Autodesk Inventor part; units mm, degrees
ref_plane "YZ Plane" through (0, 0, 0) normal (1, 0, 0) x (0, 1, 0)
ref_plane "XZ Plane" through (0, 0, 0) normal (0, 1, 0) x (-1, 0, 0)
ref_plane "XY Plane" through (0, 0, 0) normal (0, 0, 1) x (1, 0, 0)
sketch "Sketch1" plane through (0, 0, 0) normal (0, 0, 1) x (1, 0, 0)
  line L0 (-28, 11) -> (28, 11)
  line L1 (28, 11) -> (28, 9)
  line L2 (28, 9) -> (-28, 9)
  line L3 (-28, 9) -> (-28, 11)
  line L4 (-27, -7) -> (27, -7)
  line L5 (27, -7) -> (27, -9)
  line L6 (27, -9) -> (-27, -9)
  line L7 (-27, -9) -> (-27, -7)
  line L8 (-20, 1.5) -> (20, 1.5)
  line L9 (20, 1.5) -> (20, -1.5)
  line L10 (20, -1.5) -> (-20, -1.5)
  line L11 (-20, -1.5) -> (-20, 1.5)
  line L12 (26.5, 11) -> (27.8333, 15)
  line L13 (27.8333, 15) -> (29.3333, 15)
  line L14 (29.3333, 15) -> (29.3333, 4.5)
  line L15 (29.3333, 4.5) -> (22.8333, 0)
  line L16 (22.8333, 0) -> (29, -6.1667)
  line L17 (29, -6.1667) -> (29, -13)
  line L18 (29, -13) -> (27.5, -13)
  line L19 (27.5, -13) -> (25.5, -9)
  line L20 (20, -1.5) -> (25.5, -7)
  line L21 (26.5, 9) -> (28, 9)
  line L22 (28, 9) -> (28, 11)
  line L23 (28, 11) -> (26.5, 11)
  line L24 (26.5, 9) -> (26.5, 6)
  line L25 (26.5, 6) -> (20, 1.5)
  point P0 (0, 0)
  point P1 (0, 9)
  point P2 (0, -7)
  point P3 (0, -1.5)
  point P4 (20, 0)
  dimension "d0" = 2
  dimension "d1" = 2
  dimension "d2" = 56
  dimension "d3" = 54
  dimension "d4" = 7
  dimension "d6" = 3
  dimension "d7" = 40
  dimension "d8" = 1.5
  dimension "d9" = 1.5
  dimension "d10" = 1.5
  dimension "d11" = 1.5
  dimension "d13" = 2
  dimension "d14" = 1.5
  dimension "d16" = 4
  dimension "d17" = 4
  dimension "d18" = 1.5
  dimension "d26" = 3
  dimension "d28" = 15
extrude "Extrusion1" add sketch "Sketch1" along normal blind 7 contours L12 L13 L14 L15 L16 L17 L18 L19 L6 L5 L4 L20 L9 L25 L24 L2 L1 L0
mirror "Mirror1" about plane through (0, 0, 0) normal (1, 0, 0) of "Extrusion1"
sketch "Sketch2" plane through (0, 0, 0) normal (0, 0, 1) x (1, 0, 0)
  line L0 (-20, 1.5) -> (-20, -1.5)
  line L1 (20, 1.5) -> (20, -1.5)
  line L2 (-20, 1.5) -> (20, 1.5)
  line L3 (20, 1.5) -> (20, -1.5)
  line L4 (20, -1.5) -> (-20, -1.5)
  line L5 (-20, -1.5) -> (-20, 1.5)
  point P0 (0, 0)
extrude "Extrusion2" add sketch "Sketch2" along normal up to surface (7 mm away)
fillet "Fillet1" radius 2 6 edges at (22.8333, 0, 3.5) (-22.8333, 0, 3.5) (-29.3333, 4.5, 3.5) (29.3333, 4.5, 3.5) (29, -6.1667, 3.5) (-29, -6.1667, 3.5)
fillet "Fillet2" radius 1 4 edges at (-26.5, 9, 3.5) (26.5, 9, 3.5) (25.5, -7, 3.5) (-25.5, -7, 3.5)
fillet "Fillet3" radius 0.5 4 edges at (-26.5, 11, 3.5) (26.5, 11, 3.5) (25.5, -9, 3.5) (-25.5, -9, 3.5)
fillet "Fillet4" radius 2 2 edges at (26.5, 6, 3.5) (-26.5, 6, 3.5)
properties part number "conector-rpi-arduino-improved"
Read the model definition and answer for the solid it produces. Units are mm, in the model's axes. A direction names the side the tool comes from. Give positions to 0.01 mm unless a question says otherwise; leave off trailing zeros. Write each loop counter-clockwise with the first axis right and the second up, starting at its lowest first coordinate (ties: lowest second). Pieces come first, ordered by that corner, then holes. Notation, with made-up numbers: (40, 40) -> (96, 40) arc R35 ccw to (96, 77) -> close; hole circle Ø3 at (37.5, -34). An arc over 180 degrees is marked (long way). Answer in a Markdown table with one row per item.
1) Section B-B on x = -11 is taken. Give the vertices of the cut face in (y, z).
Results list:
| item | result |
|---|---|
| outline | (-1.5, 0) -> (1.5, 0) -> (1.5, 7) -> (-1.5, 7) -> close |
2) Section C-C on x = -21.5 is taken. Give the vertices of the cut face in (y, z), plus the area to 3 significant figures.
Results list:
| item | result |
|---|---|
| outline | (-3, 0) -> (2.54, 0) -> (2.54, 7) -> (-3, 7) -> close |
| area | 38.8 mm^2 |
3) Determine the mould class of faces 1 (the flat face through (26.444, -3.611, 3.451)), 2 (the flat face through (29.333, 10, 3)), 3 (the flat face through (-27.3, 13.4, 3.5)) for opening direction Y: released by +Y, released by -Y, zero draft, split by the parting line, or undercut.
Results list:
| item | result |
|---|---|
| face 1 | undercut |
| face 2 | zero draft |
| face 3 | released by +Y |
4) A tool of negligible diameter and unlimited length cuts with its end or side. For faces 4 (the flat face through (0, -1.5, 3)), 5 (the flat face through (-26.498, -3.665, 3.451)), 6 (the flat face through (-29, -10, 3)), from which of +Z, -Z, +X, -X, +Y, -Y can it reach the whole face along a straight path? Write none if from no direction.
Results list:
| item | result |
|---|---|
| face 4 | +Z, -Z, -Y |
| face 5 | +Z, -Z, -X |
| face 6 | +Z, -Z, -X, -Y |
5) Each of these flat-tipped pins is pushed along its axis until it touches: pin 1 Ø12 at (x, y) = (18, -2.5) entering from -Z; pin 2 Ø1.2 at (x, z) = (26, 3) entering from -Y; pin 3 Ø1.6 at (y, z) = (-8.5, 2) entering from -X; pin 4 Ø0.5 at (x, z) = (-26.5, 3.5) entering from -Y. Where does it stop, or does it pass through?
Results list:
| item | result |
|---|---|
| pin 1 | z = 0 |
| pin 2 | y = -11.2 |
| pin 3 | x = -29 |
| pin 4 | y = -11.5 |
6) Section A-A on y = -4.5 is taken. Give the vertices of the cut face in (x, z), plus the area to 3 significant figures.
Results list:
| item | result |
|---|---|
| outline | (-27.33, 0) -> (-23, 0) -> (-23, 7) -> (-27.33, 7) -> close; (23, 0) -> (27.33, 0) -> (27.33, 7) -> (23, 7) -> close |
| area | 60.7 mm^2 |
7) Straight lines are drawn through the part: line 1 (Y direction, x = -26, z = 1.25); line 2 (Y direction, x = -16.5, z = 4.75); line 3 (X direction, y = -11, z = 5.5). For each, find the intervals that lie inside material, in ascending order. Write a range as [from, to].
Results list:
| item | result |
|---|---|
| line 1 | [-10, -9.11], [-7, -3.17], [2.19, 5.73] |
| line 2 | [-1.5, 1.5] |
| line 3 | [-29, -26.5], [26.5, 29] |
